```python
from build123d import *

# Parameters (mm, degrees)
F0_W     = 60
F0_H     = 40
F0_R     = 8.260965
F2_DEPTH = 25.4


with BuildPart() as f2:
    # F0 (on Top) → F2 (new body)
    with BuildSketch(Plane.XY):
        Rectangle(F0_W, F0_H)
        with BuildLine():
            ThreePointArc((-25, 12), (-27.12132, 17.12132), (-22, 15))
            Line((-22, 15), (22, 15))
            ThreePointArc((22, 15), (25, 18), (28, 15))
            ThreePointArc((28, 15), (27.12132, 12.87868), (25, 12))
            Line((25, 12), (25, -12))
            ThreePointArc((25, -12), (27.12132, -12.87868), (28, -15))
            ThreePointArc((28, -15), (25, -18), (22, -15))
            Line((22, -15), (-22, -15))
            ThreePointArc((-22, -15), (-27.12132, -17.12132), (-25, -12))
            Line((-25, -12), (-25, 12))
        make_face(mode=Mode.SUBTRACT)
        with BuildLine():
            Line((22, 15), (-22, 15))
            ThreePointArc((-22, 15), (-22.87868, 12.87868), (-25, 12))
            Line((-25, 12), (-25, -12))
            ThreePointArc((-25, -12), (-22.87868, -12.87868), (-22, -15))
            Line((-22, -15), (22, -15))
            ThreePointArc((22, -15), (22.87868, -12.87868), (25, -12))
            Line((25, -12), (25, 12))
            ThreePointArc((25, 12), (22.87868, 12.87868), (22, 15))
        make_face()
        Circle(F0_R, mode=Mode.SUBTRACT)
    extrude(amount=F2_DEPTH)


solid = f2.part
```
Can you work these out from the model? Positions are in its coordinate system, mm. Coordinates: 2 decimals unless noted, no trailing zeros. Loops run counter-clockwise (first coordinate to the right, second up) from the corner with the lowest first, then second, coordinate; pieces in that order, holes last. Notation, with made-up numbers: (22, 19.25) -> (76, 19.25) arc R23 ccw to (76, 47.25) -> close; hole circle Ø3 at (-27.75, 61.5). An arc over 180 degrees is marked (long way). Put each result on its own line as item: value. Start each with the question number.
Q1. Thinking about a two-plate mould opening in Y: for faces 1 (the face through (-1.08, 8.19, 12.52)), 2 (the face through (0, -20, 13)), 3 (the face through (-7, 5, 25.4)), which applies, pulls with the +Y half, pulls with the -Y half, needs draft (parallel to the pull), parting line crosses it, or undercut?
Q2. If I drill on line 1 (Y direction, x = -25, z = 9); line 2 (X direction, y = 15, z = 19); line 3 (Y direction, x = 23.5, z = 23.25), over which ranges is the centre line in solid material (lowest first)? Write a range as [from, to].
Q3. I want a section at B-B (y = 0). Write out the boundary of the cut face in (x, z), plus the area to 3 significant figures.
Q4. I want a section at A-A (x = 0). Write out the boundary of the cut face in (y, z), plus the area to 3 significant figures.
Q5. I want a section at C-C (z = 23.75). Write out the boundary of the cut face in (x, y).
Taken from the geometry:
1. face 1: undercut
1. face 2: pulls with the -Y half
1. face 3: needs draft
2. line 1: y = [-20, -18], [-12, 12], [18, 20]
2. line 2: x = [-30, -28], [-22, 22], [28, 30]
2. line 3: y = [-20, -17.6], [-12.4, 12.4], [17.6, 20]
3. outline: (-30, 0) -> (-8.26, 0) -> (-8.26, 25.4) -> (-30, 25.4) -> close; (8.26, 0) -> (30, 0) -> (30, 25.4) -> (8.26, 25.4) -> close
3. area: 1,100 mm2
4. outline: (-20, 0) -> (-8.26, 0) -> (-8.26, 25.4) -> (-20, 25.4) -> close; (8.26, 0) -> (20, 0) -> (20, 25.4) -> (8.26, 25.4) -> close
4. area: 596 mm2
5. outline: (-30, -20) -> (30, -20) -> (30, 20) -> (-30, 20) -> close; hole (-25, -12) arc R3 ccw (long way) to (-22, -15) arc R3 ccw to start; hole (-25, 12) arc R3 ccw to (-22, 15) arc R3 ccw (long way) to start; hole circle Ø16.52 at (0, 0); hole (22, -15) arc R3 ccw to (28, -15) arc R3 ccw to (25, -12) arc R3 ccw to start; hole (22, 15) arc R3 ccw to (25, 12) arc R3 ccw to (28, 15) arc R3 ccw to start
